Can you work these out from the model? Positions are in its coordinate system, mm. A direction names the side the tool comes from. Give positions to 0.01 mm unless a question says otherwise; leave off trailing zeros. Order: outer loops, then holes, each group sorted by start corner. A loop starts at its lowest first (then second) coordinate and runs counter-clockwise, first axis right, second up.
Item 1: I'm going to push flat-ended pins straight in: pin 1 Ø2.5 at (x, z) = (14.75, 4.85) entering from +Y; pin 2 Ø3.5 at (x, z) = (15.5, -4.5) entering from +Y; pin 3 Ø1 at (x, y) = (-24.5, 14) entering from +Z; pin 4 Ø1.5 at (x, y) = (10.5, 42.5) entering from +Z. Where does each tip first touch, or does it pass through?
Item 2: I want a section at B-B, the plane x = 0. Count the separate pieces of the cut face and the enclosed holes in it, then the cut area to 3 significant figures.
Item 3: I want a section at C-C, the plane z = 19.5. Write out the boundary of the cut face in (x, y), then the cut area to 3 significant figures.
Item 4: Which directions (+Z, -Z, +X, -X, +Y, -Y) give clear straight access to the entire face, cutting with the end or side of a thin tool? Please do faces 1 (the flat face through (12, 11, -6)), 2 (the flat face through (-30.39, 25.35, 18.81)), 3 (the flat face through (22, 40, -3.641)).
Item 5: If we mould it in two halves opening along X, with no side actions, what happens to faces 4 (the flat face through (-36, 10, 1)), 5 (the flat face through (-14, 0, 0)), 6 (the flat face through (-53.125, 25, 0))? For each: +X half, -X half, draft (parallel to the pull), parting line (faces both ways), or undercut.
Item 6: I want a section at D-D, the plane x = 14.75. Write out the boundary of the cut face in (y, z), then the cut area to 3 significant figures.
Item 7: I want a section at A-A, the plane x = -34.75. Write out the boundary of the cut face in (y, z), then the cut area to 3 significant figures.
Item 8: If I drill on line 1 along X through (y, z) = (6, 4) (3 decimals); line 2 along X through (y, z) = (28, -7) (1 decimal); line 3 along Y through (x, z) = (6.5, 8), over which ranges is the centre line in solid material (lowest first)?
```python
from build123d import *

# Parameters (mm, degrees)
BOSS_EXTRUDE1_DEPTH       = 40
REVOLVE1_START            = -44.95139953
REVOLVE1_OUTLINE_R        = 13.5
REVOLVE1_DEPTH            = 30.829897511
M18_CLEARANCE_HOLE1_D     = 20
M18_CLEARANCE_HOLE1_DEPTH = 25
SKETCH9_W                 = 1.6
SKETCH9_H                 = 27
CUT_EXTRUDE4_DEPTH        = 76.299241718
CUT_EXTRUDE4_DEPTH_BACK   = 76.299241718
SKETCH18_R                = 1.6
SCALE2_SCALE              = 1.25
SKETCH19_W                = 57
SKETCH19_H                = 20
CUT_EXTRUDE5_DEPTH        = 39
SKETCH20_W                = 40
SKETCH20_H                = 20
CUT_EXTRUDE6_DEPTH        = 10
SKETCH21_R                = 5.5
CUT_EXTRUDE7_DEPTH        = 96.0605556
SKETCH22_W                = 7.783449774
SKETCH22_H                = 2
SKETCH22_W_2              = 10.366550226
CUT_EXTRUDE8_DEPTH        = 2
SKETCH23_W                = 9.71853625
SKETCH23_H                = 7.281011564
CUT_EXTRUDE9_DEPTH        = 20
SKETCH25_W                = 2.5
SKETCH25_H                = 9
BOSS_EXTRUDE3_DEPTH       = 10
SKETCH26_W                = 2.5
SKETCH26_H                = 2
BOSS_EXTRUDE4_DEPTH       = 8
SKETCH27_R                = 2.1
CUT_EXTRUDE10_DEPTH       = 8


with BuildPart() as part:
    # Sketch1 → Boss-Extrude1 (new body)
    with BuildSketch(Plane(origin=(0, 40, 0), x_dir=(1, 0, 0), z_dir=(0, 1, 0))):
        with BuildLine():
            Line((-5.61521172, 20.235350191), (-42.5, 10))
            Line((-42.5, 10), (-42.5, -10))
            Line((-42.5, -10), (-5.61521172, -20.235350191))
            ThreePointArc((-5.61521172, -20.235350191), (21, 0), (-5.61521172, 20.235350191))
        make_face()
    extrude(amount=-BOSS_EXTRUDE1_DEPTH)

    # Revolve1: read off the stored shape, not the designer's step
    # Revolve1 outline → Revolve1 (add)
    with BuildSketch(Plane(origin=(0, 0, 0), x_dir=(0.9799247046208294, -0.02083962380947531, -0.19827577601224947), z_dir=(0.19936793441719802, 0.10243002349202102, 0.9745565745577031)).offset(REVOLVE1_START)):
        with Locations((-1.9070974, 22.005607966)):
            Circle(REVOLVE1_OUTLINE_R)
    extrude(amount=REVOLVE1_DEPTH)

    # M18 Clearance Hole1
    with Locations(Plane(origin=(-8.961867673, -4.60437291, -43.807681948), x_dir=(-0.9799247046208296, 0.02083962380947534, 0.19827577601224922), z_dir=(-0.19936793441719777, -0.10243002349202121, -0.9745565745577032))):
        with Locations((1.9070974, 22.005607966)):
            Hole(M18_CLEARANCE_HOLE1_D / 2, depth=M18_CLEARANCE_HOLE1_DEPTH)

    # Sketch9 → M3.5 Clearance Hole1 (revolve, cut)
    with BuildSketch(Plane(origin=(-18.009225855, 18.806465846, -31.591069121), x_dir=(-0.12392681772022805, 0.7153744254872676, -0.6876638533531477), z_dir=(0.1561720753640579, 0.6984304843277114, 0.6984304843277114))):
        with Locations((0.8, 13.5)):
            Rectangle(SKETCH9_W, SKETCH9_H)
    revolve(axis=Axis((-11.78670398, 18.674134235, -32.850120299), (-0.9799247046208297, 0.020839623809475325, 0.19827577601224802)), mode=Mode.SUBTRACT)

    # Sketch18 → Cut-Extrude4 (cut, two sides: drawn at the far end of the back side and taken through both)
    with BuildSketch(Plane(origin=(-1.740210315, 0.03700828, 0.352110268), x_dir=(-0.19823095447813932, 0.004215689735382395, -0.9801462730872066), z_dir=(0.9799247046208297, -0.020839623809475356, -0.19827577601224802)).offset(-CUT_EXTRUDE4_DEPTH_BACK)):
        with Locations(Location((34.613136918, 18.419306886, 0), (0, 0, 359.758405588))):
            Circle(SKETCH18_R)
    extrude(amount=CUT_EXTRUDE4_DEPTH + CUT_EXTRUDE4_DEPTH_BACK, mode=Mode.SUBTRACT)


with BuildPart() as part_1:
    # Scale2: scaled about (0, 0, 0)
    add(part.part.scale(SCALE2_SCALE))

    # Sketch19 → Cut-Extrude5 (cut)
    with BuildSketch(Plane(origin=(0, 50, 0), x_dir=(1, 0, 0), z_dir=(0, 1, 0))):
        with Locations((-11.2875, 0)):
            Rectangle(SKETCH19_W, SKETCH19_H)
    extrude(amount=-CUT_EXTRUDE5_DEPTH, mode=Mode.SUBTRACT)

    # Sketch20 → Cut-Extrude6 (cut)
    with BuildSketch(Plane(origin=(0, 11, 0), x_dir=(1, 0, 0), z_dir=(0, 1, 0))):
        with Locations((-13.154050226, 0)):
            Rectangle(SKETCH20_W, SKETCH20_H)
    extrude(amount=-CUT_EXTRUDE6_DEPTH, mode=Mode.SUBTRACT)

    # Sketch21 → Cut-Extrude7 (cut, through all)
    with BuildSketch(Plane.XZ):
        with Locations(Location((0, 0, 0), (0, 0, 270))):
            Circle(SKETCH21_R)
    extrude(amount=-CUT_EXTRUDE7_DEPTH, mode=Mode.SUBTRACT)

    # Sketch22 → Cut-Extrude8 (cut)
    with BuildSketch(Plane(origin=(0, 11, 0), x_dir=(1, 0, 0), z_dir=(0, 1, 0))):
        with Locations((-37.045775113, 0)):
            Rectangle(SKETCH22_W, SKETCH22_H)
        with Locations((12.029224887, 0)):
            Rectangle(SKETCH22_W_2, SKETCH22_H)
    extrude(amount=-CUT_EXTRUDE8_DEPTH, mode=Mode.SUBTRACT)

    # Sketch23 → Cut-Extrude9 (cut)
    with BuildSketch(Plane(origin=(0, 50, 0), x_dir=(1, 0, 0), z_dir=(0, 1, 0))):
        with Locations((22.071768125, 0)):
            Rectangle(SKETCH23_W, SKETCH23_H)
    extrude(amount=-CUT_EXTRUDE9_DEPTH, mode=Mode.SUBTRACT)

    # Sketch25 → Boss-Extrude3 (add)
    with BuildSketch(Plane(origin=(0, 1, 0), x_dir=(1, 0, 0), z_dir=(0, 1, 0))):
        with Locations((-31.904050226, 5.5)):
            Rectangle(SKETCH25_W, SKETCH25_H)
        with Locations((-31.904050226, -5.5)):
            Rectangle(SKETCH25_W, SKETCH25_H)
    extrude(amount=BOSS_EXTRUDE3_DEPTH)

    # Sketch26 → Boss-Extrude4 (add)
    with BuildSketch(Plane(origin=(0, 1, 0), x_dir=(1, 0, 0), z_dir=(0, 1, 0))):
        with Locations((-31.904050226, 0)):
            Rectangle(SKETCH26_W, SKETCH26_H)
    extrude(amount=BOSS_EXTRUDE4_DEPTH)

    # Sketch27 → Cut-Extrude10 (cut)
    with BuildSketch(Plane(origin=(0, 11, 0), x_dir=(1, 0, 0), z_dir=(0, 1, 0))):
        with Locations(Location((14.75, 4.85, 0), (0, 0, 270))):
            Circle(SKETCH27_R)
        with Locations(Location((14.75, -4.85, 0), (0, 0, 270))):
            Circle(SKETCH27_R)
        with Locations(Location((-34.75, 4.85, 0), (0, 0, 270))):
            Circle(SKETCH27_R)
        with Locations(Location((-34.75, -4.85, 0), (0, 0, 270))):
            Circle(SKETCH27_R)
    extrude(amount=-CUT_EXTRUDE10_DEPTH, mode=Mode.SUBTRACT)


solid = part_1.part
```
Results list:
1. pin 1: stops at y = 3
1. pin 2: stops at y = 50
1. pin 3: stops at z = 20.58
1. pin 4: stops at z = 24.37
2. separate pieces: 2
2. enclosed holes: 1
2. area: 2,160 mm2
3. outline: (-27.9, 0) - (17.57, 0) - (17.57, 50) - (-27.9, 50) - close
3. area: 2,270 mm2
4. face 1: +Y
4. face 2: +Z, -X, +Y, -Y
4. face 3: +X, +Y
5. face 4: undercut
5. face 5: draft
5. face 6: -X half
6. outline: (0, -21.71) - (50, -21.71) - (50, -10) - (11, -10) - (11, -6.95) - (3, -6.95) - (3, -2.75) - (11, -2.75) - (11, -1) - (9, -1) - (9, 1) - (11, 1) - (11, 2.75) - (3, 2.75) - (3, 6.95) - (11, 6.95) - (11, 10) - (50, 10) - (50, 21.71) - (0, 21.71) - close
6. area: 1,320 mm2
7. outline: (0, -17.6) - (50, -17.6) - (50, -10) - (11, -10) - (11, -6.95) - (3, -6.95) - (3, -2.75) - (11, -2.75) - (11, -1) - (9, -1) - (9, 1) - (11, 1) - (11, 2.75) - (3, 2.75) - (3, 6.95) - (11, 6.95) - (11, 10) - (50, 10) - (50, 17.6) - (0, 17.6) - close
7. area: 909 mm2
8. line 1: x = -53.125 to -36.67, -32.83 to -30.654, 6.846 to 12.83, 16.67 to 25.943
8. line 2: x = -53.1 to -39.8, 17.2 to 25.3
8. line 3: y = 0 to 1
